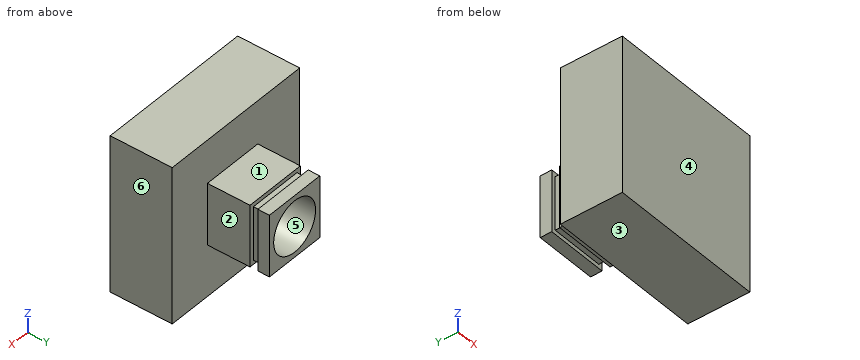
Autodesk Inventor part; units mm, degrees
ref_plane "YZ Plane" through (0, 0, 0) normal (1, 0, 0) x (0, 1, 0)
ref_plane "XZ Plane" through (0, 0, 0) normal (0, 1, 0) x (-1, 0, 0)
ref_plane "XY Plane" through (0, 0, 0) normal (0, 0, 1) x (1, 0, 0)
sketch "Sketch1" plane through (0, 0, 0) normal (0, 1, 0) x (-1, 0, 0)
  line L0 (0, 0) -> (76, 0)
  line L1 (76, 0) -> (76, -76)
  line L2 (76, -76) -> (0, -76)
  line L3 (0, -76) -> (0, 0)
  dimension "d0" = 76
  dimension "d1" = 76
extrude "Extrusion1" add sketch "Sketch1" along normal blind 30
sketch "Sketch2" plane through (0, 30, 0) normal (0, 1, 0) x (1, 0, 0)
  point P0 (0, 0)
sketch "Sketch3" plane through (0, 30, 0) normal (0, 1, 0) x (1, 0, 0)
  line L0 (-51, 21) -> (-21, 21)
  line L1 (-21, 21) -> (-21, 51)
  line L2 (-21, 51) -> (-51, 51)
  line L3 (-51, 51) -> (-51, 21)
  point P0 (0, 0)
  dimension "d4" = 30
  dimension "d5" = 30
extrude "Extrusion2" add sketch "Sketch3" along normal blind 30
sketch "Sketch4" plane through (-21, 30, -21) normal (1, 0, 0) x (0, 0, -1)
  line L0 (30, 0) -> (30, 30)
  line L1 (0, 20.6) -> (30, 20.6)
  line L2 (30, 20.6) -> (30, 24.4)
  line L3 (30, 24.4) -> (0, 24.4)
  line L4 (0, 24.4) -> (0, 20.6)
  point P0 (-21, -30)
  point P1 (0, 22.5)
  point P2 (30, 22.5)
  dimension "d8" = 3.8
sketch "Sketch5" plane through (-21, 30, -51) normal (0, 0, -1) x (-1, 0, 0)
  line L0 (30, 0) -> (30, 30)
  line L1 (0, 20.6) -> (30, 20.6)
  line L2 (30, 20.6) -> (30, 24.4)
  line L3 (30, 24.4) -> (0, 24.4)
  line L4 (0, 24.4) -> (0, 20.6)
  line L5 (0, 20.6) -> (30, 24.4) construction
  line L6 (30, 20.6) -> (0, 24.4) construction
  point P0 (-21, -30)
  point P1 (30, 22.5)
  point P2 (15, 22.5)
  dimension "d9" = 3.8
sketch "Sketch6" plane through (-51, 30, -51) normal (-1, 0, 0) x (0, 0, 1)
  line L0 (30, 0) -> (30, 30)
  line L1 (0, 20.6) -> (30, 20.6)
  line L2 (30, 20.6) -> (30, 24.4)
  line L3 (30, 24.4) -> (0, 24.4)
  line L4 (0, 24.4) -> (0, 20.6)
  line L5 (0, 20.6) -> (30, 24.4) construction
  line L6 (30, 20.6) -> (0, 24.4) construction
  point P0 (51, -30)
  point P1 (15, 22.5)
  dimension "d10" = 3.8
sketch "Sketch7" plane through (-51, 30, -21) normal (0, 0, 1) x (1, 0, 0)
  line L0 (30, 0) -> (30, 30)
  line L1 (0, 24.4) -> (30, 24.4)
  line L2 (30, 24.4) -> (30, 20.6)
  line L3 (30, 20.6) -> (0, 20.6)
  line L4 (0, 20.6) -> (0, 24.4)
  line L5 (0, 24.4) -> (30, 20.6) construction
  line L6 (30, 24.4) -> (0, 20.6) construction
  point P0 (51, -30)
  point P1 (15, 22.5)
  dimension "d11" = 3.8
extrude "Extrusion3" cut sketch "Sketch6" against normal blind 2
extrude "Extrusion4" cut sketch "Sketch7" against normal blind 2
extrude "Extrusion5" cut sketch "Sketch4" against normal blind 2
extrude "Extrusion6" cut sketch "Sketch5" against normal blind 2
sketch "Sketch8" plane through (0, 60, 0) normal (0, 1, 0) x (1, 0, 0)
  line L0 (-21, 21) -> (-51, 21)
  line L1 (-21, 51) -> (-21, 21)
  circle A0 centre (-36, 36) radius 12.5
  point P0 (0, 0)
  dimension "d20" = 25
extrude "Extrusion7" cut sketch "Sketch8" against normal blind 25
properties part number "Hydraulic cylinder part 1.dwg"
Verification items for the finished model (mm, model axes). Face numbers are marked on the shaded views. A direction names the side the tool comes from. Coordinates: 2 decimals unless noted, no trailing zeros. Order: outer loops, then holes, each group sorted by start corner. A loop starts at its lowest first (then second) coordinate and runs counter-clockwise, first axis right, second up. Notation, with made-up numbers: (40.5, 75) -> (72.5, 75) arc R21 cw to (72.5, 109) -> close; hole circle Ø8 at (51.5, 6). An arc over 180 degrees is marked (long way). Put each result on its own line as item: value. Start each with the question number.
1. Mould release check, pull along X, two halves, no side actions. Record for the marked faces 4, 5 and 6: released by +X, released by -X, zero draft, split by the parting line, or undercut.
2. Go/stop test with flat-tipped pins: pin 1 Ø15 at (x, z) = (-36, -36) entering from +Y; pin 2 Ø12 at (x, z) = (-61, -46) entering from +Y; pin 3 Ø1.5 at (y, z) = (48.5, -44.5) entering from +X. Record where each tip stops, or that it passes through.
3. Cross-section at C-C, the plane x = -36. Record the boundary of the cut face in (y, z).
4. Cross-section at D-D, the plane y = 31. Record the boundary of the cut face in (x, z), then the cut area to 3 significant figures.
5. Access from +Z, -Z, +X, -X, +Y, -Y to the whole of each face (thin tool, end or side, straight path). Record for the marked faces 1, 2 and 3.
6. Cross-section at B-B, the plane z = -36. Record the boundary of the cut face in (x, y).
7. Cross-section at A-A, the plane y = 45. Record the boundary of the cut face in (x, z), then the cut area to 3 significant figures.
8. Material ranges on L1, parallel to X at y = 45.5, z = -36; L2, parallel to X at y = 52.75, z = -36, recorded low to high. Write a range as [from, to].
Computed:
1. face 4: zero draft
1. face 5: undercut
1. face 6: released by +X
2. pin 1: y = 35
2. pin 2: y = 30
2. pin 3: x = -21
3. outline: (0, -76) -> (30, -76) -> (30, -51) -> (50.6, -51) -> (50.6, -49) -> (54.4, -49) -> (54.4, -51) -> (60, -51) -> (60, -48.5) -> (35, -48.5) -> (35, -23.5) -> (60, -23.5) -> (60, -21) -> (54.4, -21) -> (54.4, -23) -> (50.6, -23) -> (50.6, -21) -> (30, -21) -> (30, 0) -> (0, 0) -> close
4. outline: (-51, -51) -> (-21, -51) -> (-21, -21) -> (-51, -21) -> close
4. area: 900 mm2
5. face 1: +Z, +X, -X, +Y
5. face 2: +Z, -Z, +X, +Y
5. face 3: -Z, +X, -X, +Y, -Y
6. outline: (-76, 0) -> (0, 0) -> (0, 30) -> (-21, 30) -> (-21, 50.6) -> (-23, 50.6) -> (-23, 54.4) -> (-21, 54.4) -> (-21, 60) -> (-23.5, 60) -> (-23.5, 35) -> (-48.5, 35) -> (-48.5, 60) -> (-51, 60) -> (-51, 54.4) -> (-49, 54.4) -> (-49, 50.6) -> (-51, 50.6) -> (-51, 30) -> (-76, 30) -> close
7. outline: (-51, -51) -> (-21, -51) -> (-21, -21) -> (-51, -21) -> close; hole circle Ø25 at (-36, -36)
7. area: 409 mm2
8. L1: [-51, -48.5], [-23.5, -21]
8. L2: [-49, -48.5], [-23.5, -23]
